Study the drawing (mm; zero at the part's minimum x, y, z) and answer. A direction names the side the tool comes from. Coordinates: 2 decimals unless noted, no trailing zeros. Put each result on its own line as item: value.
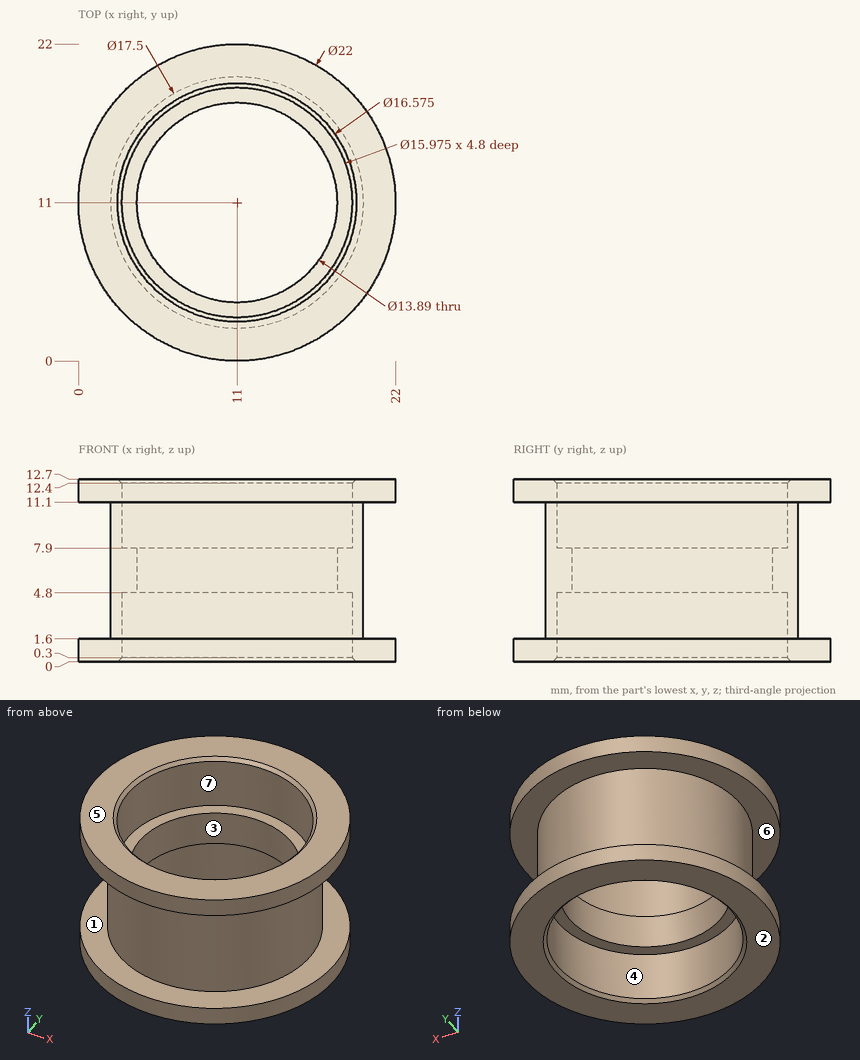
Q1. Consider line 1 along Z through (x, y) = (1.5, 11.25); line 2 along X through (y, z) = (11, 11.35); line 3 along X through (y, z) = (11, 7.1) (3 decimals). Determine where each line is inside the solid, lowest interval first.
Answers below:
line 1: z = 0 to 1.6, 11.1 to 12.7
line 2: x = 0 to 3.01, 18.99 to 22
line 3: x = 2.25 to 4.055, 17.945 to 19.75
Q2. A tool of negligible diameter and unlimited length cuts with its end or side. For the marked faces 4, 5, 6 and 7, from which of +Z, -Z, +X, -X, +Y, -Y can it reach the whole face along a straight path? Write none if from no direction.
Answers below:
face 4: -Z
face 5: +Z, +X, -X, +Y, -Y
face 6: none
face 7: +Z
Q3. Given pin 1 (6.5 mm diameter, centred on x = 15, y = 14, fed in from +Z); pin 2 (3 mm diameter, centred on y = 10, z = 5.5, fed in from -X); pin 3 (2 mm diameter, centred on x = 9.5, z = 9, fed in from +Y), each flat-ended and moving along its own axis, determine where each tip first touches the part or whether it passes through.
Answers below:
pin 1: stops at z = 12.66
pin 2: stops at x = 2.25
pin 3: stops at y = 19.74
Q4. For a pull along Z with two mould halves and no side action, classify the marked faces 1, 2 and 3 as +Z half, -Z half, draft (parallel to the pull), parting line (faces both ways), or undercut.
Answers below:
face 1: undercut
face 2: -Z half
face 3: draft
